from build123d import *

# Parameters (mm, degrees)
F1_DEPTH = 10
F3_DEPTH = 4
F4_W     = 5.5
F4_H     = 11.188021542
F4_H_2   = 22.7246312633
F4_H_3   = 10.0103956625
F5_DEPTH = 25
F6_DEPTH = 4
F8_D     = 4
F8_DEPTH = 9
F8_TIP   = 1.2017212381


# Not quite as in the source:
# - a feature names something its author has since deleted; it is built from what else it names


with BuildPart() as f1:
    # F0 (on Top) → F1 (new body)
    with BuildSketch(Plane.XY):
        Polygon((60, 11.5470053838), (40, 46.1880215352), (-40, 46.1880215352), (-60, 11.5470053838), (-20, -57.735026919), (20, -57.735026919), align=None)
    extrude(amount=F1_DEPTH)

    # F2 (on face) → F3 (cut)
    with BuildSketch(Plane.XY.offset(10)):
        Polygon((-42.8867513499, 31.188021542), (-48.4529946241, 21.5470053838), (-5.5662432742, -52.7350269258), (5.5662432742, -52.7350269258), (48.4529946241, 21.5470053838), (42.8867513499, 31.188021542), align=None)
    extrude(amount=-F3_DEPTH, mode=Mode.SUBTRACT)

    # F4 (on face) + F1_face (on face) → F5 (cut)
    with BuildSketch(Plane.XY.offset(6)):
        with BuildLine():
            ThreePointArc((-5.5, -10.6653645039), (-12, 0), (-5.5, 10.6653645039))
            Line((-5.5, 10.6653645039), (-5.5, 20))
            Line((-5.5, 20), (-5.5, 31.188021542))
            Line((-5.5, 31.188021542), (-42.8867513499, 31.188021542))
            Line((-42.8867513499, 31.188021542), (-48.4529946241, 21.5470053838))
            Line((-48.4529946241, 21.5470053838), (-11.3457479046, -42.7246312633))
            Line((-11.3457479046, -42.7246312633), (-5.5, -42.7246312633))
            Line((-5.5, -42.7246312633), (-5.5, -20))
            Line((-5.5, -20), (-5.5, -10.6653645039))
        make_face()
        with Locations((2.75, 25.594010771)):
            Rectangle(F4_W, F4_H)
        with Locations((-2.75, 25.594010771)):
            Rectangle(F4_W, F4_H)
        with BuildLine():
            ThreePointArc((-5.5, 10.6653645039), (-2.8298079399, 11.6615688063), (0, 12))
            Line((0, 12), (0, 20))
            Line((0, 20), (-5.5, 20))
            Line((-5.5, 20), (-5.5, 10.6653645039))
        make_face()
        with BuildLine():
            ThreePointArc((-5.5, 5.8094750193), (-2.9600844452, 7.4322204002), (0, 8))
            Line((0, 8), (0, 12))
            ThreePointArc((0, 12), (-2.8298079399, 11.6615688063), (-5.5, 10.6653645039))
            Line((-5.5, 10.6653645039), (-5.5, 5.8094750193))
        make_face()
        with BuildLine():
            ThreePointArc((-5.5, 2.3979157617), (-3.2872865277, 5.0193373352), (0, 6))
            Line((0, 6), (0, 8))
            ThreePointArc((0, 8), (-2.9600844452, 7.4322204002), (-5.5, 5.8094750193))
            Line((-5.5, 5.8094750193), (-5.5, 2.3979157617))
        make_face()
        with BuildLine():
            Line((5.5, -2.3979157617), (5.5, 2.3979157617))
            ThreePointArc((5.5, 2.3979157617), (3.2872865277, 5.0193373352), (0, 6))
            ThreePointArc((0, 6), (-3.2872865277, 5.0193373352), (-5.5, 2.3979157617))
            Line((-5.5, 2.3979157617), (-5.5, -2.3979157617))
            ThreePointArc((-5.5, -2.3979157617), (-3.2872865277, -5.0193373352), (0, -6))
            ThreePointArc((0, -6), (3.2872865277, -5.0193373352), (5.5, -2.3979157617))
        make_face()
        with BuildLine():
            ThreePointArc((-5.5, -2.3979157617), (-6, 0), (-5.5, 2.3979157617))
            Line((-5.5, 2.3979157617), (-5.5, 5.8094750193))
            ThreePointArc((-5.5, 5.8094750193), (-8, 0), (-5.5, -5.8094750193))
            Line((-5.5, -5.8094750193), (-5.5, -2.3979157617))
        make_face()
        with BuildLine():
            ThreePointArc((-5.5, -5.8094750193), (-8, 0), (-5.5, 5.8094750193))
            Line((-5.5, 5.8094750193), (-5.5, 10.6653645039))
            ThreePointArc((-5.5, 10.6653645039), (-12, 0), (-5.5, -10.6653645039))
            Line((-5.5, -10.6653645039), (-5.5, -5.8094750193))
        make_face()
        with BuildLine():
            Line((-5.5, -2.3979157617), (-5.5, 2.3979157617))
            ThreePointArc((-5.5, 2.3979157617), (-6, 0), (-5.5, -2.3979157617))
        make_face()
        with BuildLine():
            Line((0, -8), (0, -6))
            ThreePointArc((0, -6), (-3.2872865277, -5.0193373352), (-5.5, -2.3979157617))
            Line((-5.5, -2.3979157617), (-5.5, -5.8094750193))
            ThreePointArc((-5.5, -5.8094750193), (-2.9600844452, -7.4322204002), (0, -8))
        make_face()
        with BuildLine():
            Line((0, -12), (0, -8))
            ThreePointArc((0, -8), (-2.9600844452, -7.4322204002), (-5.5, -5.8094750193))
            Line((-5.5, -5.8094750193), (-5.5, -10.6653645039))
            ThreePointArc((-5.5, -10.6653645039), (-2.8298079399, -11.6615688063), (0, -12))
        make_face()
        with BuildLine():
            Line((0, -20), (0, -12))
            ThreePointArc((0, -12), (-2.8298079399, -11.6615688063), (-5.5, -10.6653645039))
            Line((-5.5, -10.6653645039), (-5.5, -20))
            Line((-5.5, -20), (0, -20))
        make_face()
        with Locations((-2.75, -31.3623156317)):
            Rectangle(F4_W, F4_H_2)
        with Locations((2.75, -31.3623156317)):
            Rectangle(F4_W, F4_H_2)
        with BuildLine():
            Line((5.5, 20), (5.5, 10.6653645039))
            ThreePointArc((5.5, 10.6653645039), (10.246950766, 6.2449979984), (12, 0))
            ThreePointArc((12, 0), (10.246950766, -6.2449979984), (5.5, -10.6653645039))
            Line((5.5, -10.6653645039), (5.5, -20))
            Line((5.5, -20), (5.5, -42.7246312633))
            Line((5.5, -42.7246312633), (11.3457479046, -42.7246312633))
            Line((11.3457479046, -42.7246312633), (48.4529946241, 21.5470053838))
            Line((48.4529946241, 21.5470053838), (42.8867513499, 31.188021542))
            Line((42.8867513499, 31.188021542), (5.5, 31.188021542))
            Line((5.5, 31.188021542), (5.5, 20))
        make_face()
        Polygon((11.3457479046, -42.7246312633), (5.5, -42.7246312633), (5.5, -52.7350269258), (5.5662432742, -52.7350269258), align=None)
        with Locations((2.75, -47.7298290946)):
            Rectangle(F4_W, F4_H_3)
        with Locations((-2.75, -47.7298290946)):
            Rectangle(F4_W, F4_H_3)
        Polygon((-5.5, -52.7350269258), (-5.5, -42.7246312633), (-11.3457479046, -42.7246312633), (-5.5662432742, -52.7350269258), align=None)
        with BuildLine():
            ThreePointArc((5.5, -2.3979157617), (5.8736700622, -1.2247448714), (6, 0))
            ThreePointArc((6, 0), (5.8736700622, 1.2247448714), (5.5, 2.3979157617))
            Line((5.5, 2.3979157617), (5.5, -2.3979157617))
        make_face()
    with BuildSketch(Plane.XY.offset(10)):
        Polygon((60, 11.5470053838), (40, 46.1880215352), (-40, 46.1880215352), (-60, 11.5470053838), (-20, -57.735026919), (20, -57.735026919), align=None)
        Polygon((-48.4529946241, 21.5470053838), (-42.8867513499, 31.188021542), (42.8867513499, 31.188021542), (48.4529946241, 21.5470053838), (5.5662432742, -52.7350269258), (-5.5662432742, -52.7350269258), align=None, mode=Mode.SUBTRACT)
    extrude(amount=-F5_DEPTH, mode=Mode.SUBTRACT)

    # F4 (on face) → F6 (join)
    with BuildSketch(Plane.XY.offset(6)):
        with BuildLine():
            ThreePointArc((0, 12), (2.8298079399, 11.6615688063), (5.5, 10.6653645039))
            Line((5.5, 10.6653645039), (5.5, 20))
            Line((5.5, 20), (0, 20))
            Line((0, 20), (0, 12))
        make_face()
        with BuildLine():
            ThreePointArc((0, 8), (2.9600844452, 7.4322204002), (5.5, 5.8094750193))
            Line((5.5, 5.8094750193), (5.5, 10.6653645039))
            ThreePointArc((5.5, 10.6653645039), (2.8298079399, 11.6615688063), (0, 12))
            Line((0, 12), (0, 8))
        make_face()
        with BuildLine():
            Line((5.5, 10.6653645039), (5.5, 5.8094750193))
            ThreePointArc((5.5, 5.8094750193), (7.3484692283, 3.1622776602), (8, 0))
            ThreePointArc((8, 0), (7.3484692283, -3.1622776602), (5.5, -5.8094750193))
            Line((5.5, -5.8094750193), (5.5, -10.6653645039))
            ThreePointArc((5.5, -10.6653645039), (10.246950766, -6.2449979984), (12, 0))
            ThreePointArc((12, 0), (10.246950766, 6.2449979984), (5.5, 10.6653645039))
        make_face()
        with BuildLine():
            Line((5.5, -10.6653645039), (5.5, -5.8094750193))
            ThreePointArc((5.5, -5.8094750193), (2.9600844452, -7.4322204002), (0, -8))
            Line((0, -8), (0, -12))
            ThreePointArc((0, -12), (2.8298079399, -11.6615688063), (5.5, -10.6653645039))
        make_face()
        with BuildLine():
            Line((5.5, -20), (5.5, -10.6653645039))
            ThreePointArc((5.5, -10.6653645039), (2.8298079399, -11.6615688063), (0, -12))
            Line((0, -12), (0, -20))
            Line((0, -20), (5.5, -20))
        make_face()
    extrude(amount=F6_DEPTH)

    # F8
    with Locations(Plane(origin=(0, 0, 0), x_dir=(0, -1, 0), z_dir=(-1, 0, 0))):
        with Locations((15, 5), (-15, 5)):
            Hole(F8_D / 2, depth=F8_DEPTH)
            with Locations((0, 0, -(F8_DEPTH + F8_TIP / 2))):  # 118° drill point
                Cone(0, F8_D / 2, F8_TIP, mode=Mode.SUBTRACT)


solid = f1.part
Geometry check sheet. Reference: the model listing, model coordinates, mm. A direction names the side the tool comes from. Give positions to 0.01 mm unless a question says otherwise; leave off trailing zeros. Loops run counter-clockwise (first coordinate to the right, second up) from the corner with the lowest first, then second, coordinate; pieces in that order, holes last. Notation, with made-up numbers: (77.5, 63) -> (95.5, 63) arc R22 cw to (95.5, 75) -> close; hole circle Ø4 at (-23, -22). An arc over 180 degrees is marked (long way). Answer in a Markdown table with one row per item. Add a question column.
1) Cross-section at C-C on z = 5. Record the boundary of the cut face in (x, y), and give its area (3 significant figures).
2) Material ranges on probe 1 along Z at (x, y) = (1.25, -15); probe 2 along Y at (x, z) = (1, 5.25); probe 3 along X at (y, z) = (13, 9.5), recorded low to high. Write a range as from..to.
3) Cross-section at B-B on y = 15. Record the boundary of the cut face in (x, z).
4) Draft check along Z on faces 4 (the face through (3, 13, 5)), 5 (the face through (6.4, -0.6, 6)), 6 (the face through (7, 0, 0)), 7 (the face through (3, -20, 5)). Enter one of: pulls with the +Z half, pulls with the -Z half, needs draft (parallel to the pull), parting line crosses it, or undercut.
5) Set-up check for faces 1 (the face through (0, 13, 4)), 2 (the face through (5.5, 17.3, 4.9)), 3 (the face through (5.5, -17.5, 4.9)): record each of +Z, -Z, +X, -X, +Y, -Y from which the full face is reachable in a straight line by a thin tool's end or side.
6) Cross-section at D-D on z = 8.25. Record the boundary of the cut face in (x, y), and give its area (3 significant figures).
7) Gauge pin test, flat ends, axial feed: P1, Ø3, axis at y = 4, z = 2, coming from the -X side; P2, Ø3, axis at y = -15.5, z = 6.5, coming from the +X side. Record the tip position at first contact, or that the pin passes through.
8) Cross-section at A-A on x = 2.25. Record the boundary of the cut face in (y, z).
Outcome:
| question | item | result |
|---|---|---|
| 1 | outline | (0, -20) -> (5.5, -20) -> (5.5, -17) -> (0, -17) -> close; (0, -13) -> (5.5, -13) -> (5.5, -10.67) arc R12 ccw to (5.5, 10.67) -> (5.5, 13) -> (0, 13) -> (0, 6) arc R6 cw to (0, -6) -> close; (0, 17) -> (5.5, 17) -> (5.5, 20) -> (0, 20) -> close |
| 1 | area | 218 mm^2 |
| 2 | probe 1 | z = 0..3, 7..10 |
| 2 | probe 2 | y = -20..-16.98, -13.02..-5.92, 5.92..13.02, 16.98..20 |
| 2 | probe 3 | x = 0..5.5 |
| 3 | outline | (0, 0) -> (5.5, 0) -> (5.5, 3) -> (0, 3) -> close; (0, 7) -> (5.5, 7) -> (5.5, 10) -> (0, 10) -> close |
| 4 | face 4 | undercut |
| 4 | face 5 | pulls with the +Z half |
| 4 | face 6 | pulls with the -Z half |
| 4 | face 7 | needs draft |
| 5 | face 1 | +Z, -Z, -X, +Y, -Y |
| 5 | face 2 | +Z, -Z, +X, +Y |
| 5 | face 3 | +Z, -Z, +X, -Y |
| 6 | outline | (0, -20) -> (5.5, -20) -> (5.5, -10.67) arc R12 ccw to (5.5, 10.67) -> (5.5, 20) -> (0, 20) -> (0, 8) arc R8 cw to (0, -8) -> close |
| 6 | area | 218 mm^2 |
| 7 | P1 | stops at x = 2.4 |
| 7 | P2 | stops at x = 5.5 |
| 8 | outline | (-20, 0) -> (-5.56, 0) -> (-5.56, 6) -> (-7.68, 6) -> (-7.68, 10) -> (-20, 10) -> close; (5.56, 0) -> (20, 0) -> (20, 10) -> (7.68, 10) -> (7.68, 6) -> (5.56, 6) -> close; hole circle Ø4 at (-15, 5); hole circle Ø4 at (15, 5) |
